Can you work these out from the model? Positions are in its coordinate system, mm. Face numbers are marked on the shaded views. A direction names the side the tool comes from. Round coordinates to 2 decimals unless told otherwise and drop trailing zeros. Loops run counter-clockwise (first coordinate to the right, second up) from the corner with the lowest first, then second, coordinate; pieces in that order, holes last. Notation, with made-up numbers: (39, -3) -> (47, -3) arc R24 ccw to (47, 16) -> close; hole circle Ø7 at (-16, 35.5). An arc over 180 degrees is marked (long way). Use a Markdown table: item, result.
from build123d import *

# Parameters (mm, degrees)
SKETCH1_R           = 5
BOSS_EXTRUDE1_DEPTH = 30
SKETCH3_R           = 1.5
CUT_EXTRUDE1_DEPTH  = 6
SKETCH5_R           = 9.45
BOSS_EXTRUDE2_DEPTH = 2


with BuildPart() as part:
    # Sketch1 → Boss-Extrude1 (new body)
    with BuildSketch(Plane.XY):
        with BuildLine():
            Line((-40, 15), (40, 15))
            ThreePointArc((40, 15), (45.476992863, -13.964331319), (29.802327604, 11.00033989))
            Line((29.802327604, 11.00033989), (-29.802327604, 11.00033989))
            ThreePointArc((-29.802327604, 11.00033989), (-45.476992863, -13.964331319), (-40, 15))
        make_face()
        with Locations((-40, 0)):
            Circle(SKETCH1_R, mode=Mode.SUBTRACT)
        with Locations((40, 0)):
            Circle(SKETCH1_R, mode=Mode.SUBTRACT)
    extrude(amount=BOSS_EXTRUDE1_DEPTH)

    # Sketch3 → Cut-Extrude1 (cut)
    with BuildSketch(Plane(origin=(0, 15, 0), x_dir=(1, 0, 0), z_dir=(0, 1, 0))):
        with Locations(Location((-22.15, -15, 0), (0, 0, 270))):
            Circle(SKETCH3_R)
        with Locations(Location((22.15, -15, 0), (0, 0, 270))):
            Circle(SKETCH3_R)
    extrude(amount=-CUT_EXTRUDE1_DEPTH, mode=Mode.SUBTRACT)

    # Sketch5 → Boss-Extrude2 (add)
    with BuildSketch(Plane.XY.offset(30)):
        with Locations((-40, 0)):
            Circle(SKETCH5_R)
        with Locations((40, 0)):
            Circle(SKETCH5_R)
    extrude(amount=-BOSS_EXTRUDE2_DEPTH)


solid = part.part
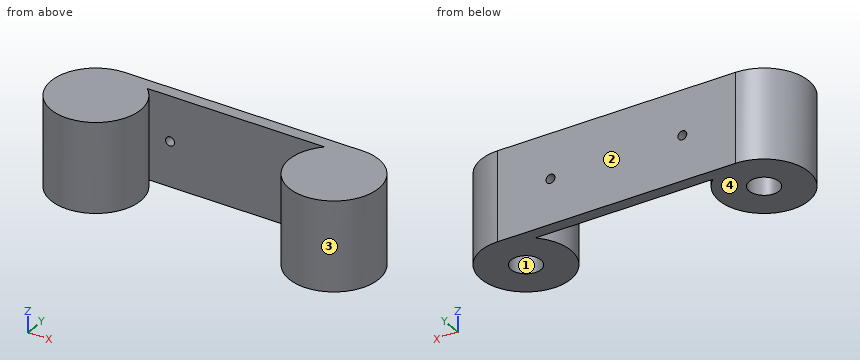
1. I want a section at C-C (x = -22.15). Please give me the cut outline in (y, z), plus the area to 3 significant figures.
Answer sheet:
| item | result |
|---|---|
| outline | (11, 0) -> (15, 0) -> (15, 13.5) -> (11, 13.5) -> close; (11, 16.5) -> (15, 16.5) -> (15, 30) -> (11, 30) -> close |
| area | 108 mm² |
2. If we mould it in two halves opening along X, with no side actions, what happens to the marked faces 3 and 4? For each: +X half, -X half, draft (parallel to the pull), parting line (faces both ways), or undercut.
Answer sheet:
| item | result |
|---|---|
| face 3 | undercut |
| face 4 | draft |
3. Will these pins go through, and if not, where does the flat tip stop? pin 1 Ø3 at (y, z) = (10.5, 7) entering from -X; pin 2 Ø3 at (x, z) = (-44, 7) entering from -Y; pin 3 Ø4 at (x, z) = (-22.15, 15) entering from -Y.
Answer sheet:
| item | result |
|---|---|
| pin 1 | stops at x = -52 |
| pin 2 | stops at y = -14.79 |
| pin 3 | stops at y = 11 |
4. I need wall thicknesses on line 1 (X direction, y = 0, z = 22); line 2 (Z direction, x = -22, y = 12); line 3 (Y direction, x = -40, z = 19.5). Which ranges of each line are inside material? Lowest first, please.
Answer sheet:
| item | result |
|---|---|
| line 1 | x = -55 to -45, -35 to -25, 25 to 35, 45 to 55 |
| line 2 | z = 0 to 13.51, 16.49 to 30 |
| line 3 | y = -15 to -5, 5 to 15 |
5. I want a section at A-A (z = 15). Please give me the cut outline in (x, y).
Answer sheet:
| item | result |
|---|---|
| outline | (-40, 15) arc R15 ccw (long way) to (-29.8, 11) -> (-23.65, 11) -> (-23.65, 15) -> close; (-20.65, 11) -> (20.65, 11) -> (20.65, 15) -> (-20.65, 15) -> close; (23.65, 11) -> (29.8, 11) arc R15 ccw (long way) to (40, 15) -> (23.65, 15) -> close; hole circle Ø10 at (-40, 0); hole circle Ø10 at (40, 0) |
6. I want a section at B-B (y = 0). Please give me the cut outline in (x, z), plus the area to 3 significant figures.
Answer sheet:
| item | result |
|---|---|
| outline | (-55, 0) -> (-45, 0) -> (-45, 28) -> (-35, 28) -> (-35, 0) -> (-25, 0) -> (-25, 30) -> (-55, 30) -> close; (25, 0) -> (35, 0) -> (35, 28) -> (45, 28) -> (45, 0) -> (55, 0) -> (55, 30) -> (25, 30) -> close |
| area | 1,240 mm² |
7. Which directions (+Z, -Z, +X, -X, +Y, -Y) give clear straight access to the entire face, cutting with the end or side of a thin tool? Please do the marked faces 1 and 2.
Answer sheet:
| item | result |
|---|---|
| face 1 | -Z |
| face 2 | +Z, -Z, +X, -X, +Y |
8. I want a section at D-D (z = 4.25). Please give me the cut outline in (x, y).
Answer sheet:
| item | result |
|---|---|
| outline | (-40, 15) arc R15 ccw (long way) to (-29.8, 11) -> (29.8, 11) arc R15 ccw (long way) to (40, 15) -> close; hole circle Ø10 at (-40, 0); hole circle Ø10 at (40, 0) |
